Build history of the part. All positions in model axes, mm. A direction names the side the tool comes from. Give positions to 0.01 mm unless a question says otherwise; leave off trailing zeros. Write each loop counter-clockwise with the first axis right and the second up, starting at its lowest first coordinate (ties: lowest second). Pieces come first, ordered by that corner, then holes. Notation, with made-up numbers: M 1.5,49.25 L 20.5,49.25 A24 ccw 20.5,76.25 Z; hole C -26.75,4.25 d10. An arc over 180 degrees is marked long. Return JSON: item names as keys, results as strings. Group by question number.
Q1. Flat gauge pins, fed straight in: pin 1 Ø10 at (x, y) = (57.5, 163.5) entering from -Z; pin 2 Ø1 at (x, z) = (105, 0.5) entering from +Y; pin 3 Ø1.3 at (x, z) = (94.5, 0.5) entering from -Y. Where does each tip first touch, or does it go through?
Q2. Band-saw the part on B-B, the plane z = -19. Give the cut face in (x, y), then the cut area to 3 significant figures.
Q3. Wall check: probe 1 along Y at (x, z) = (74.5, 0.5); probe 2 along Z at (x, y) = (64, 34); probe 3 along X at (y, z) = (177.5, -32). Give the ranges that are in metal, low to high.
Q4. Pull direction Y, two halves, no side cores. Call faces 1 (the cylindrical face through (9.1, 34.3, 0.6)), 2 (the flat face through (-5.633, 103, -19)): +Y half, -Y half, draft (parallel to the pull), parting line (faces both ways), or undercut.
Q5. Band-saw the part on A-A, the plane y = 51. Give the cut face in (x, z).
Q6. Tool access for faces 3 (the flat face through (51, 127, 0)), 4 (the cylindrical face through (12.77, 174.71, 0.61)): list every direction of +Z, -Z, +X, -X, +Y, -Y with a clear straight run to the whole face (end or side of a thin tool).
from build123d import *

# Parameters (mm, degrees)
SKETCH2_W           = 113.00010125
SKETCH2_H           = 190.5995575
SKETCH2_R           = 2.1
SKETCH2_R_2         = 1.85
BOSS_EXTRUDE1_DEPTH = 1.2
SKETCH5_W           = 2
SKETCH5_H           = 37.6
SKETCH5_H_2         = 0.6
CUT_EXTRUDE2_DEPTH  = 2.2
CUT_EXTRUDE1_DEPTH  = 2.2
SKETCH9_W           = 14
SKETCH9_H           = 3.4
SKETCH9_W_2         = 8.5
BOSS_EXTRUDE5_DEPTH = 1.2
FILLET1_R           = 1
CUT_EXTRUDE4_REACH  = 3.2
SKETCH10_W          = 8.2
SKETCH10_H          = 0.7
SKETCH11_R          = 2.25
CUT_EXTRUDE5_DEPTH  = 2.2
BOSS_EXTRUDE6_DEPTH = 1.2
SKETCH13_R          = 1.635773904
CUT_EXTRUDE6_DEPTH  = 2.2
SKETCH14_W          = 1.2
SKETCH14_H          = 152.3995575
BOSS_EXTRUDE7_DEPTH = 32
BOSS_EXTRUDE8_DEPTH = 1.2
BOSS_EXTRUDE9_DEPTH = 1.2
CUT_EXTRUDE7_REACH  = 117.2
FILLET2_R           = 1


with BuildPart() as part:
    # Sketch2 → Boss-Extrude1 (new body)
    with BuildSketch(Plane.XY):
        with Locations((49.667238625, 126.88082875)):
            Rectangle(SKETCH2_W, SKETCH2_H)
        with Locations((8.16763175, 151.180160625)):
            Circle(SKETCH2_R, mode=Mode.SUBTRACT)
        with Locations((100.1668405, 151.180160625)):
            Circle(SKETCH2_R_2, mode=Mode.SUBTRACT)
        with Locations((100.1668405, 36.181495)):
            Circle(SKETCH2_R_2, mode=Mode.SUBTRACT)
        with Locations((8.16763175, 36.181495)):
            Circle(SKETCH2_R, mode=Mode.SUBTRACT)
    extrude(amount=BOSS_EXTRUDE1_DEPTH)

    # Sketch5 → Cut-Extrude2 (cut, through all)
    with BuildSketch(Plane.XY.offset(1.2)):
        Polygon((-4.832812, 185.1806075), (5.667188, 185.1806075), (5.667188, 222.1806075), (-6.832812, 222.1806075), (-6.832812, 185.1806075), (-6.832812, 184.5806075), (-4.832812, 184.5806075), align=None)
        with Locations((105.16728925, 203.3806075)):
            Rectangle(SKETCH5_W, SKETCH5_H)
        with Locations((-5.832812, 31.88105)):
            Rectangle(SKETCH5_W, SKETCH5_H_2)
        with Locations((105.16728925, 31.88105)):
            Rectangle(SKETCH5_W, SKETCH5_H_2)
    extrude(amount=-CUT_EXTRUDE2_DEPTH, mode=Mode.SUBTRACT)

    # Sketch4 → Cut-Extrude1 (cut, through all)
    with BuildSketch(Plane.XY.offset(1.2)):
        with BuildLine():
            Line((55.16728925, 218.1806075), (98.16728925, 218.1806075))
            ThreePointArc((98.16728925, 218.1806075), (99.581502812, 217.594821062), (100.16728925, 216.1806075))
            Line((100.16728925, 216.1806075), (100.16728925, 192.1806075))
            ThreePointArc((100.16728925, 192.1806075), (99.581502812, 190.766393938), (98.16728925, 190.1806075))
            Line((98.16728925, 190.1806075), (55.16728925, 190.1806075))
            ThreePointArc((55.16728925, 190.1806075), (53.753075688, 190.766393938), (53.16728925, 192.1806075))
            Line((53.16728925, 192.1806075), (53.16728925, 216.1806075))
            ThreePointArc((53.16728925, 216.1806075), (53.753075688, 217.594821062), (55.16728925, 218.1806075))
        make_face()
    extrude(amount=-CUT_EXTRUDE1_DEPTH, mode=Mode.SUBTRACT)

    # Sketch9 → Boss-Extrude5 (add)
    with BuildSketch(Plane.XY.offset(1.2)):
        with Locations((4.167188, 29.88105)):
            Rectangle(SKETCH9_W, SKETCH9_H)
        with Locations((96.16728925, 29.88105)):
            Rectangle(SKETCH9_W, SKETCH9_H)
        with Locations((50.167238625, 29.88105)):
            Rectangle(SKETCH9_W, SKETCH9_H)
        with Locations((1.417188, 186.8806075)):
            Rectangle(SKETCH9_W_2, SKETCH9_H)
    extrude(amount=-BOSS_EXTRUDE5_DEPTH)

    # Fillet1
    fillet1_edges = [part.edges().sort_by_distance(p)[0] for p in [
        (103.16728925, 28.18105, 0.6),
        (89.16728925, 28.18105, 0.6),
        (57.167238625, 28.18105, 0.6),
        (43.167238625, 28.18105, 0.6),
        (11.167188, 28.18105, 0.6),
        (-2.832812, 28.18105, 0.6),
        (-2.832812, 188.5806075, 0.6),
    ]]
    fillet(fillet1_edges, radius=FILLET1_R)

    # Sketch10 → Cut-Extrude4 (cut, up to next)
    with BuildSketch(Plane.XY.offset(1.2), mode=Mode.PRIVATE) as cut_extrude4_sk1:
        with Locations((96.16728925, 31.93105)):
            Rectangle(SKETCH10_W, SKETCH10_H)
    cut_extrude4_tool1 = extrude(cut_extrude4_sk1.sketch, amount=-CUT_EXTRUDE4_REACH, mode=Mode.PRIVATE) & part.part
    add(cut_extrude4_tool1.solids().sort_by_distance((96.167289, 31.93105, 1.2))[0], mode=Mode.SUBTRACT)
    # Sketch10 → Cut-Extrude4 (cut, up to next)
    with BuildSketch(Plane.XY.offset(1.2), mode=Mode.PRIVATE) as cut_extrude4_sk2:
        with Locations((50.167238625, 31.93105)):
            Rectangle(SKETCH10_W, SKETCH10_H)
    cut_extrude4_tool2 = extrude(cut_extrude4_sk2.sketch, amount=-CUT_EXTRUDE4_REACH, mode=Mode.PRIVATE) & part.part
    add(cut_extrude4_tool2.solids().sort_by_distance((50.167239, 31.93105, 1.2))[0], mode=Mode.SUBTRACT)
    # Sketch10 → Cut-Extrude4 (cut, up to next)
    with BuildSketch(Plane.XY.offset(1.2), mode=Mode.PRIVATE) as cut_extrude4_sk3:
        with Locations((4.167188, 31.93105)):
            Rectangle(SKETCH10_W, SKETCH10_H)
    cut_extrude4_tool3 = extrude(cut_extrude4_sk3.sketch, amount=-CUT_EXTRUDE4_REACH, mode=Mode.PRIVATE) & part.part
    add(cut_extrude4_tool3.solids().sort_by_distance((4.167188, 31.93105, 1.2))[0], mode=Mode.SUBTRACT)
    # Sketch10 → Cut-Extrude4 (cut, up to next)
    with BuildSketch(Plane.XY.offset(1.2), mode=Mode.PRIVATE) as cut_extrude4_sk4:
        with Locations((50.167238625, 184.8306075)):
            Rectangle(SKETCH10_W, SKETCH10_H)
    cut_extrude4_tool4 = extrude(cut_extrude4_sk4.sketch, amount=-CUT_EXTRUDE4_REACH, mode=Mode.PRIVATE) & part.part
    add(cut_extrude4_tool4.solids().sort_by_distance((50.167239, 184.830607, 1.2))[0], mode=Mode.SUBTRACT)
    # Sketch10 → Cut-Extrude4 (cut, up to next)
    with BuildSketch(Plane.XY.offset(1.2), mode=Mode.PRIVATE) as cut_extrude4_sk5:
        with Locations((96.16728925, 184.8306075)):
            Rectangle(SKETCH10_W, SKETCH10_H)
    cut_extrude4_tool5 = extrude(cut_extrude4_sk5.sketch, amount=-CUT_EXTRUDE4_REACH, mode=Mode.PRIVATE) & part.part
    add(cut_extrude4_tool5.solids().sort_by_distance((96.167289, 184.830607, 1.2))[0], mode=Mode.SUBTRACT)
    # Sketch10 → Cut-Extrude4 (cut, up to next)
    with BuildSketch(Plane.XY.offset(1.2), mode=Mode.PRIVATE) as cut_extrude4_sk6:
        with Locations((4.167188, 184.8306075)):
            Rectangle(SKETCH10_W, SKETCH10_H)
    cut_extrude4_tool6 = extrude(cut_extrude4_sk6.sketch, amount=-CUT_EXTRUDE4_REACH, mode=Mode.PRIVATE) & part.part
    add(cut_extrude4_tool6.solids().sort_by_distance((4.167188, 184.830607, 1.2))[0], mode=Mode.SUBTRACT)

    # Sketch11 → Cut-Extrude5 (cut, through all)
    with BuildSketch(Plane.XY.offset(1.2)):
        with Locations((61.367697375, 160.67994375)):
            Circle(SKETCH11_R)
        with Locations((13.067697375, 172.47994375)):
            Circle(SKETCH11_R)
        with BuildLine():
            Line((71.867697375, 175.27994375), (71.867697375, 170.27994375))
            ThreePointArc((71.867697375, 170.27994375), (69.367697375, 167.77994375), (66.867697375, 170.27994375))
            Line((66.867697375, 170.27994375), (66.867697375, 175.27994375))
            ThreePointArc((66.867697375, 175.27994375), (69.367697375, 177.77994375), (71.867697375, 175.27994375))
        make_face()
    extrude(amount=-CUT_EXTRUDE5_DEPTH, mode=Mode.SUBTRACT)

    # Sketch12 → Boss-Extrude6 (add)
    with BuildSketch(Plane.XY.offset(1.2)):
        with BuildLine():
            Line((104.16728925, 222.1806075), (104.16728925, 213.7806075))
            ThreePointArc((104.16728925, 213.7806075), (108.36728925, 217.9806075), (104.16728925, 222.1806075))
        make_face()
    extrude(amount=-BOSS_EXTRUDE6_DEPTH)

    # Sketch13 → Cut-Extrude6 (cut, through all)
    with BuildSketch(Plane.XY.offset(1.2)):
        with Locations((104.16728925, 217.9806075)):
            Circle(SKETCH13_R)
        with Locations((47.16728925, 217.9806075)):
            Circle(SKETCH13_R)
        with Locations((9.667188, 217.9806075)):
            Circle(SKETCH13_R)
    extrude(amount=-CUT_EXTRUDE6_DEPTH, mode=Mode.SUBTRACT)

    # Sketch14 → Boss-Extrude7 (add)
    with BuildSketch(Plane(origin=(0, 0, 0), x_dir=(-1, 0, 0), z_dir=(0, 0, -1))):
        with Locations((6.232812, 108.38082875)):
            Rectangle(SKETCH14_W, SKETCH14_H)
    extrude(amount=BOSS_EXTRUDE7_DEPTH)

    # Sketch16 → Boss-Extrude8 (add)
    with BuildSketch(Plane.ZY.offset(6.832812)):
        with BuildLine():
            Line((-32, 32.18105), (-4, 32.18105))
            ThreePointArc((-4, 32.18105), (-6.121320344, 31.302370344), (-7, 29.18105))
            Line((-7, 29.18105), (-7, 18.18105))
            Line((-7, 18.18105), (-32, 18.18105))
            Line((-32, 18.18105), (-32, 32.18105))
        make_face()
    extrude(amount=-BOSS_EXTRUDE8_DEPTH)

    # Sketch17 → Boss-Extrude9 (add)
    with BuildSketch(Plane.ZY.offset(6.832812)):
        with BuildLine():
            Line((-32, 184.5806075), (-38, 184.5806075))
            Line((-38, 184.5806075), (-38, 168.5806075))
            Line((-38, 168.5806075), (-35, 168.5806075))
            ThreePointArc((-35, 168.5806075), (-32.878679656, 167.701927844), (-32, 165.5806075))
            Line((-32, 165.5806075), (-32, 184.5806075))
        make_face()
    extrude(amount=-BOSS_EXTRUDE9_DEPTH)

    # Sketch15 → Cut-Extrude7 (cut, up to next)
    with BuildSketch(Plane.ZY.offset(6.832812), mode=Mode.PRIVATE) as cut_extrude7_sk1:
        with BuildLine():
            Line((-46.8, 177.7806075), (-34.8, 177.7806075))
            ThreePointArc((-34.8, 177.7806075), (-33.2, 176.1806075), (-34.8, 174.5806075))
            Line((-34.8, 174.5806075), (-46.8, 174.5806075))
            ThreePointArc((-46.8, 174.5806075), (-48.4, 176.1806075), (-46.8, 177.7806075))
        make_face()
    cut_extrude7_tool1 = extrude(cut_extrude7_sk1.sketch, amount=-CUT_EXTRUDE7_REACH, mode=Mode.PRIVATE) & part.part
    add(cut_extrude7_tool1.solids().sort_by_distance((-6.832812, 176.180608, -40.8))[0], mode=Mode.SUBTRACT)
    # Sketch15 → Cut-Extrude7 (cut, up to next)
    with BuildSketch(Plane.ZY.offset(6.832812), mode=Mode.PRIVATE) as cut_extrude7_sk2:
        with BuildLine():
            Line((-25.1, 21.18105), (-25.1, 18.18105))
            Line((-25.1, 18.18105), (-21.9, 18.18105))
            Line((-21.9, 18.18105), (-21.9, 21.18105))
            ThreePointArc((-21.9, 21.18105), (-23.5, 22.78105), (-25.1, 21.18105))
        make_face()
    cut_extrude7_tool2 = extrude(cut_extrude7_sk2.sketch, amount=-CUT_EXTRUDE7_REACH, mode=Mode.PRIVATE) & part.part
    add(cut_extrude7_tool2.solids().sort_by_distance((-6.832812, 20.324349, -23.5))[0], mode=Mode.SUBTRACT)

    # Fillet2
    fillet2_edges = [part.edges().sort_by_distance(p)[0] for p in [
        (5.667188, 222.1806075, 0.6),
        (-6.232812, 18.18105, -32),
        (-6.232812, 18.18105, -7),
        (-6.232812, 168.5806075, -38),
        (-6.232812, 184.5806075, -38),
    ]]
    fillet(fillet2_edges, radius=FILLET2_R)


solid = part.part
From the geometry:
{
 "1": {"pin 1": "stops at z = 0", "pin 2": "stops at y = 222.17", "pin 3": "stops at y = 28.18"},
 "2": {"outline": "M -6.83,18.18 L -5.63,18.18 L -5.63,184.58 L -6.83,184.58 Z", "area": "200 mm^2"},
 "3": {"probe 1": "y = 31.58 to 190.18, 218.18 to 222.18", "probe 2": "z = 0 to 1.2", "probe 3": "x = -6.83 to -5.63"},
 "4": {"face 1": "undercut", "face 2": "draft"},
 "5": {"outline": "M -6.83,-32 L -5.63,-32 L -5.63,0 L 106.17,0 L 106.17,1.2 L -6.83,1.2 Z"},
 "6": {"face 3": "-Z, +X, +Y, -Y", "face 4": "+Z, -Z"}
}
